Part model, mm, in its own coordinate system. A direction names the side the tool comes from. Coordinates: 2 decimals unless noted, no trailing zeros. Write each loop counter-clockwise with the first axis right and the second up, starting at its lowest first coordinate (ties: lowest second). Pieces come first, ordered by that corner, then holes. Notation, with made-up numbers: M 13.25,11.5 L 24.25,11.5 A7 ccw 24.25,23.5 Z; hole C 83.5,1 d9. An arc over 180 degrees is marked long. Use a Markdown table: item, result. Add a question column.
Q1. Slice it at A-A on z = 63. Write the cut outline in (x, y), then the cut area to 3 significant figures.
Q2. Tool access for faces 1 (the flat face through (151, 6, -37.1)), 2 (the cylindrical face through (154.08, 6.26, 1.22)), 3 (the flat face through (-151, 6, 87.9)), 4 (the cylindrical face through (-107.188, 0.493, 58.784)), 5 (the flat face through (157.5, 6, -106)): list every direction of +Z, -Z, +X, -X, +Y, -Y with a clear straight run to the whole face (end or side of a thin tool).
Q3. Pin check, flat tip, straight feed: pin 1 Ø4 at (y, z) = (7, 54) entering from -X. Stop position of the tip, or through.
Q4. Wall check: L1, parallel to X at y = 7, z = 0 (3 decimals); L2, parallel to Z at x = 151.15, y = 5.5 (3 decimals); L3, parallel to X at y = 7.75, z = -40. Give the ranges that are in metal, low to high. Write a range as from..to.
Q5. Mould opens along X. For faces 6 (the flat face through (-2, 6, 125)), 7 (the cylindrical face through (-149.7, 6.3, 118.3)), 8 (the flat face through (-157.5, 6, 107)), 9 (the flat face through (144.8, 6, -62)) say: released by +X, released by -X, zero draft, split by the parting line, or undercut.
Q6. Slice it at B-B on z = -46. Write the cut outline in (x, y), then the cut area to 3 significant figures.
from build123d import *

# Parameters (mm, degrees)
CROQUIS1_W              = 315
CROQUIS1_H              = 250
CROQUIS1_R              = 3.175
SALIENTE_EXTRUIR1_DEPTH = 12.7
CROQUIS2_W              = 12.7
CROQUIS2_H              = 50.8
CORTAR_EXTRUIR1_DEPTH   = 13.7
CROQUIS3_R              = 5
CORTAR_EXTRUIR2_DEPTH   = 1


with BuildPart() as part:
    # Croquis1 → Saliente-Extruir1 (new body)
    with BuildSketch(Plane(origin=(0, 0, 0), x_dir=(1, 0, 0), z_dir=(0, 1, 0))):
        Rectangle(CROQUIS1_W, CROQUIS1_H)
        with Locations((-151.15, -115.475)):
            Circle(CROQUIS1_R, mode=Mode.SUBTRACT)
        with Locations((-151.15, 0)):
            Circle(CROQUIS1_R, mode=Mode.SUBTRACT)
        with Locations((-151.15, 115.475)):
            Circle(CROQUIS1_R, mode=Mode.SUBTRACT)
        with Locations((151.15, 115.475)):
            Circle(CROQUIS1_R, mode=Mode.SUBTRACT)
        with Locations((151.15, 0)):
            Circle(CROQUIS1_R, mode=Mode.SUBTRACT)
        with Locations((151.15, -115.475)):
            Circle(CROQUIS1_R, mode=Mode.SUBTRACT)
    extrude(amount=SALIENTE_EXTRUIR1_DEPTH)

    # Croquis2 → Cortar-Extruir1 (cut, through all)
    with BuildSketch(Plane(origin=(0, 12.7, 0), x_dir=(1, 0, 0), z_dir=(0, 1, 0))):
        with Locations((-151.15, 62.5)):
            Rectangle(CROQUIS2_W, CROQUIS2_H)
        with Locations((-151.15, -62.5)):
            Rectangle(CROQUIS2_W, CROQUIS2_H)
    cortar_extruir1 = extrude(amount=-CORTAR_EXTRUIR1_DEPTH, mode=Mode.SUBTRACT)

    # Simetría1: Cortar-Extruir1 across plane
    add(cortar_extruir1.mirror(Plane(origin=(0, 0, 0), x_dir=(0, 0, 1), z_dir=(1, 0, 0))), mode=Mode.SUBTRACT)

    # Croquis3 → Cortar-Extruir2 (cut)
    with BuildSketch(Plane(origin=(0, 0, 0), x_dir=(-1, 0, 0), z_dir=(0, -1, 0))):
        with Locations((104.5, -63)):
            Circle(CROQUIS3_R)
    extrude(amount=-CORTAR_EXTRUIR2_DEPTH, mode=Mode.SUBTRACT)


solid = part.part
Recorded:
| question | item | result |
|---|---|---|
| 1 | outline | M -144.8,0 L -109.5,0 L -109.5,1 L -99.5,1 L -99.5,0 L 144.8,0 L 144.8,12.7 L -144.8,12.7 Z |
| 1 | area | 3,670 mm² |
| 2 | face 1 | +X, +Y, -Y |
| 2 | face 2 | +Y, -Y |
| 2 | face 3 | -X, +Y, -Y |
| 2 | face 4 | -Y |
| 2 | face 5 | +Z, -Z, +X, +Y, -Y |
| 3 | pin 1 | x = -144.8 |
| 4 | L1 | -157.5..-154.325, -147.975..147.975, 154.325..157.5 |
| 4 | L2 | -125..-118.65, -112.3..-87.9, -37.1..-3.175, 3.175..37.1, 87.9..112.3, 118.65..125 |
| 4 | L3 | -144.8..144.8 |
| 5 | face 6 | zero draft |
| 5 | face 7 | undercut |
| 5 | face 8 | released by -X |
| 5 | face 9 | released by +X |
| 6 | outline | M -144.8,0 L 144.8,0 L 144.8,12.7 L -144.8,12.7 Z |
| 6 | area | 3,680 mm² |
